```python
from build123d import *

# Parameters (mm, degrees)
SKETCH1_R           = 2.5
SKETCH1_R_2         = 1.75
BOSS_EXTRUDE1_DEPTH = 2.61
SKETCH2_R           = 1.75
BOSS_EXTRUDE2_DEPTH = 7.71
CUT_EXTRUDE1_START  = -2.3
CUT_EXTRUDE1_DEPTH  = 32.579406586
CUT_EXTRUDE1_TAPER  = -30
CIRPATTERN1_COUNT   = 4
CUT_EXTRUDE2_REACH  = 46.536
SKETCH6_W           = 14.35
SKETCH6_H           = 15.668786702
SKETCH7_R           = 1.75
BOSS_EXTRUDE3_DEPTH = 2
SKETCH9_W           = 16.172360651
SKETCH9_H           = 2.1
SKETCH10_R          = 6.5
SKETCH10_R_2        = 2.5
BOSS_EXTRUDE4_DEPTH = 5.3


with BuildPart() as part:
    # Sketch1 → Boss-Extrude1 (new body)
    with BuildSketch(Plane(origin=(0, 0, 0), x_dir=(1, 0, 0), z_dir=(0, 1, 0))):
        with BuildLine():
            Line((-16.375, -19.375), (16.375, -19.375))
            ThreePointArc((16.375, -19.375), (18.496320344, -18.496320344), (19.375, -16.375))
            Line((19.375, -16.375), (19.375, 16.375))
            ThreePointArc((19.375, 16.375), (18.496320344, 18.496320344), (16.375, 19.375))
            Line((16.375, 19.375), (-16.375, 19.375))
            ThreePointArc((-16.375, 19.375), (-18.496320344, 18.496320344), (-19.375, 16.375))
            Line((-19.375, 16.375), (-19.375, -16.375))
            ThreePointArc((-19.375, -16.375), (-18.496320344, -18.496320344), (-16.375, -19.375))
        make_face()
        with Locations(Location((0, 0, 0), (0, 0, 270))):
            Circle(SKETCH1_R, mode=Mode.SUBTRACT)
        with Locations(Location((-15.444979868, 15.444979868, 0), (0, 0, 270))):
            Circle(SKETCH1_R_2, mode=Mode.SUBTRACT)
        with Locations(Location((15.444979868, 15.444979868, 0), (0, 0, 270))):
            Circle(SKETCH1_R_2, mode=Mode.SUBTRACT)
        with Locations(Location((15.444979868, -15.444979868, 0), (0, 0, 270))):
            Circle(SKETCH1_R_2, mode=Mode.SUBTRACT)
        with Locations(Location((-15.444979868, -15.444979868, 0), (0, 0, 270))):
            Circle(SKETCH1_R_2, mode=Mode.SUBTRACT)
    extrude(amount=BOSS_EXTRUDE1_DEPTH)

    # Sketch2 → Boss-Extrude2 (add)
    with BuildSketch(Plane(origin=(0, 2.61, 0), x_dir=(1, 0, 0), z_dir=(0, 1, 0))):
        with BuildLine():
            Line((19.375, -16.375), (19.375, 16.375))
            ThreePointArc((19.375, 16.375), (18.496320344, 18.496320344), (16.375, 19.375))
            Line((16.375, 19.375), (-16.375, 19.375))
            ThreePointArc((-16.375, 19.375), (-18.496320344, 18.496320344), (-19.375, 16.375))
            Line((-19.375, 16.375), (-19.375, -16.375))
            ThreePointArc((-19.375, -16.375), (-18.496320344, -18.496320344), (-16.375, -19.375))
            Line((-16.375, -19.375), (16.375, -19.375))
            ThreePointArc((16.375, -19.375), (18.496320344, -18.496320344), (19.375, -16.375))
        make_face()
        with Locations(Location((-15.444979868, 15.444979868, 0), (0, 0, 270))):
            Circle(SKETCH2_R, mode=Mode.SUBTRACT)
        with Locations(Location((15.444979868, 15.444979868, 0), (0, 0, 270))):
            Circle(SKETCH2_R, mode=Mode.SUBTRACT)
        with Locations(Location((15.444979868, -15.444979868, 0), (0, 0, 270))):
            Circle(SKETCH2_R, mode=Mode.SUBTRACT)
        with Locations(Location((-15.444979868, -15.444979868, 0), (0, 0, 270))):
            Circle(SKETCH2_R, mode=Mode.SUBTRACT)
        Polygon((-7.455844123, 18), (7.455844123, 18), (18, 7.455844123), (18, -7.455844123), (7.455844123, -18), (-7.455844123, -18), (-18, -7.455844123), (-18, 7.455844123), align=None, mode=Mode.SUBTRACT)
    extrude(amount=BOSS_EXTRUDE2_DEPTH)

    # Sketch4 → Cut-Extrude1 (cut, through all)
    with BuildSketch(Plane.XZ.offset(CUT_EXTRUDE1_START)):
        with BuildLine():
            Line((12.375, 19.375), (12.375, 15.444979868))
            ThreePointArc((12.375, 15.444979868), (13.274176285, 13.274176285), (15.444979868, 12.375))
            Line((15.444979868, 12.375), (19.375, 12.375))
            Line((19.375, 12.375), (19.375, 16.375))
            ThreePointArc((19.375, 16.375), (18.496320344, 18.496320344), (16.375, 19.375))
            Line((16.375, 19.375), (12.375, 19.375))
        make_face()
    cut_extrude1 = extrude(amount=CUT_EXTRUDE1_DEPTH, taper=CUT_EXTRUDE1_TAPER, mode=Mode.SUBTRACT)

    # CirPattern1: Cut-Extrude1 ×4 about axis
    cirpattern1_axis = Axis((0, 0, 0), (0, 1, 0))
    for i in range(1, CIRPATTERN1_COUNT):
        add(cut_extrude1.rotate(cirpattern1_axis, i * 360 / CIRPATTERN1_COUNT), mode=Mode.SUBTRACT)

    # Sketch6 → Cut-Extrude2 (cut, up to next)
    with BuildSketch(Plane(origin=(19.375, 0, 0), x_dir=(0, 0, -1), z_dir=(1, 0, 0)), mode=Mode.PRIVATE) as cut_extrude2_sk1:
        with Locations((0, 12.494393351)):
            Rectangle(SKETCH6_W, SKETCH6_H)
    cut_extrude2_tool1 = extrude(cut_extrude2_sk1.sketch, amount=-CUT_EXTRUDE2_REACH, mode=Mode.PRIVATE) & part.part
    add(cut_extrude2_tool1.solids().sort_by_distance((19.375, 12.494393, 0))[0], mode=Mode.SUBTRACT)

    # Sketch7 → Boss-Extrude3 (add)
    with BuildSketch(Plane(origin=(0, 10.32, 0), x_dir=(1, 0, 0), z_dir=(0, 1, 0))):
        with BuildLine():
            Line((19.375, -7.175), (18, -7.175))
            Line((18, -7.175), (18, -7.455844123))
            Line((18, -7.455844123), (7.455844123, -18))
            Line((7.455844123, -18), (-7.455844123, -18))
            Line((-7.455844123, -18), (-18, -7.455844123))
            Line((-18, -7.455844123), (-18, 7.455844123))
            Line((-18, 7.455844123), (-7.455844123, 18))
            Line((-7.455844123, 18), (7.455844123, 18))
            Line((7.455844123, 18), (18, 7.455844123))
            Line((18, 7.455844123), (18, 7.175))
            Line((18, 7.175), (19.375, 7.175))
            Line((19.375, 7.175), (19.375, 16.375))
            ThreePointArc((19.375, 16.375), (18.496320344, 18.496320344), (16.375, 19.375))
            Line((16.375, 19.375), (-16.375, 19.375))
            ThreePointArc((-16.375, 19.375), (-18.496320344, 18.496320344), (-19.375, 16.375))
            Line((-19.375, 16.375), (-19.375, -16.375))
            ThreePointArc((-19.375, -16.375), (-18.496320344, -18.496320344), (-16.375, -19.375))
            Line((-16.375, -19.375), (16.375, -19.375))
            ThreePointArc((16.375, -19.375), (18.496320344, -18.496320344), (19.375, -16.375))
            Line((19.375, -16.375), (19.375, -7.175))
        make_face()
        with Locations(Location((-15.444979868, -15.444979868, 0), (0, 0, 90))):
            Circle(SKETCH7_R, mode=Mode.SUBTRACT)
        with Locations(Location((15.444979868, -15.444979868, 0), (0, 0, 90))):
            Circle(SKETCH7_R, mode=Mode.SUBTRACT)
        with Locations(Location((15.444979868, 15.444979868, 0), (0, 0, 90))):
            Circle(SKETCH7_R, mode=Mode.SUBTRACT)
        with Locations(Location((-15.444979868, 15.444979868, 0), (0, 0, 90))):
            Circle(SKETCH7_R, mode=Mode.SUBTRACT)
    extrude(amount=BOSS_EXTRUDE3_DEPTH)

    # Sketch9 → Cut-Revolve1 (revolve, cut)
    with BuildSketch(Plane(origin=(0, 0, 0), x_dir=(0.7071067811865475, 0, 0.7071067811865477), z_dir=(-0.7071067811865477, 0, 0.7071067811865475))):
        with Locations((14.138819675, 11.27)):
            Rectangle(SKETCH9_W, SKETCH9_H)
    revolve(axis=Axis((0, 0, 0), (0, 1, 0)), mode=Mode.SUBTRACT)

    # Sketch10 → Boss-Extrude4 (add)
    with BuildSketch(Plane(origin=(0, 2.61, 0), x_dir=(1, 0, 0), z_dir=(0, 1, 0))):
        with Locations(Location((0, 0, 0), (0, 0, 270))):
            Circle(SKETCH10_R)
        with Locations(Location((0, 0, 0), (0, 0, 270))):
            Circle(SKETCH10_R_2, mode=Mode.SUBTRACT)
    extrude(amount=BOSS_EXTRUDE4_DEPTH)


solid = part.part
```
For this review, take the finished solid that the model builds, in its own axes (mm). A direction names the side the tool comes from. Give positions to 0.01 mm unless a question says otherwise; leave off trailing zeros. Write each loop counter-clockwise with the first axis right and the second up, starting at its lowest first coordinate (ties: lowest second). Pieces come first, ordered by that corner, then holes.
Item 1: Take a section at C-C (z = 0). Give the boundary of the cut face in (x, y) (3 decimals).
Item 2: Take a section at B-B (x = 0). Give the boundary of the cut face in (y, z) (3 decimals), and give its area (3 significant figures).
Item 3: Machinability: for faces 5 (the face through (-18, 6, 0)), 6 (the face through (-17.4, 2.3, 15.9)), 7 (the face through (19, 7, -7.175)), which of the approach directions +Z, -Z, +X, -X, +Y, -Y give a long, thin tool a straight path to every point of the face, cutting with its end or side? Answer none if there is none.
Item 4: Insertion check: P1, Ø3, axis at x = 15.44, z = 15.44, coming from the -Y side; P2, Ø4, axis at x = -9.5, z = -5.5, coming from the -Y side; P3, Ø3.5, axis at x = 16.5, z = 16, coming from the -Y side; P4, Ø2, axis at x = 5, z = 5.5, coming from the +Y side. Each pin has a flat end and moves straight along its axis. Give the tip position at first contact, or say it passes through.
Item 5: Take a section at D-D (y = 3.5). Give the boundary of the cut face in (x, z) (3 decimals).
Item 6: Wall thickness on probe 1 along Z at (x, y) = (-7, 8.75) (3 decimals); probe 2 along Z at (x, y) = (-17, 10.75); probe 3 along Z at (x, y) = (10, 3) (3 decimals): over which ranges is each line inside the solid? List them lowest first.
Item 7: The part is to be moulded in two halves that separate along X. For faces 1 (the face through (17, 12.32, 17)), 2 (the face through (-18.2, 11.285, -12.756)), 3 (the face through (-8, 2.61, 0)), 4 (the face through (-18.47, 7.24, -18.52)), say which applies: +X half, -X half, draft (parallel to the pull), parting line (faces both ways), or undercut.
Item 8: Take a section at A-A (y = 6.75). Give the boundary of the cut face in (x, z) (3 decimals), and give its area (3 significant figures).
Established:
1. outline: (-19.375, 0) - (-2.5, 0) - (-2.5, 7.91) - (-6.5, 7.91) - (-6.5, 2.61) - (-18, 2.61) - (-18, 10.22) - (-19.375, 10.22) - close; (2.5, 0) - (19.375, 0) - (19.375, 4.66) - (18, 4.66) - (18, 2.61) - (6.5, 2.61) - (6.5, 7.91) - (2.5, 7.91) - close
2. outline: (0, -19.375) - (10.22, -19.375) - (10.22, -18) - (2.61, -18) - (2.61, -6.5) - (7.91, -6.5) - (7.91, -2.5) - (0, -2.5) - close; (0, 2.5) - (7.91, 2.5) - (7.91, 6.5) - (2.61, 6.5) - (2.61, 18) - (10.22, 18) - (10.22, 19.375) - (0, 19.375) - close
2. area: 151 mm2
3. face 5: +Y
3. face 6: +Z, -X, -Y
3. face 7: +X, +Y
4. P1: passes through
4. P2: stops at y = 0
4. P3: stops at y = 2.3
4. P4: stops at y = 7.91
5. outline: (-19.375, -16.375) arc R3 ccw to (-16.375, -19.375) - (16.375, -19.375) arc R3 ccw to (19.375, -16.375) - (19.375, 16.375) arc R3 ccw to (16.375, 19.375) - (-16.375, 19.375) arc R3 ccw to (-19.375, 16.375) - close; circle Ø13 at (0, 0); hole (-18, -7.456) - (-7.456, -18) - (7.456, -18) - (18, -7.456) - (18, 7.456) - (7.456, 18) - (-7.456, 18) - (-18, 7.456) - close; hole circle Ø3.5 at (-15.445, -15.445); hole circle Ø3.5 at (-15.445, 15.445); hole circle Ø5 at (0, 0); hole circle Ø3.5 at (15.445, -15.445); hole circle Ø3.5 at (15.445, 15.445)
6. probe 1: z = -19.375 to -18, 18 to 19.375
6. probe 2: z = -19.31 to -16.25, -14.64 to -14.32, 14.32 to 14.64, 16.25 to 19.31
6. probe 3: z = -19.375 to -15.456, 15.456 to 19.375
7. face 1: draft
7. face 2: undercut
7. face 3: undercut
7. face 4: -X half
8. outline: (-19.375, -16.375) arc R3 ccw to (-16.375, -19.375) - (16.375, -19.375) arc R3 ccw to (19.375, -16.375) - (19.375, -7.175) - (18, -7.175) - (18, -7.456) - (7.456, -18) - (-7.456, -18) - (-18, -7.456) - (-18, 7.456) - (-7.456, 18) - (7.456, 18) - (18, 7.456) - (18, 7.175) - (19.375, 7.175) - (19.375, 16.375) arc R3 ccw to (16.375, 19.375) - (-16.375, 19.375) arc R3 ccw to (-19.375, 16.375) - close; circle Ø13 at (0, 0); hole circle Ø3.5 at (-15.445, -15.445); hole circle Ø3.5 at (-15.445, 15.445); hole circle Ø5 at (0, 0); hole circle Ø3.5 at (15.445, -15.445); hole circle Ø3.5 at (15.445, 15.445)
8. area: 475 mm2
